Job drawing, mm, ordinate dimensions from the low corner. One solid piece. Give positions to 0.01 mm unless a question says otherwise; leave off trailing zeros. Write each loop counter-clockwise with the first axis right and the second up, starting at its lowest first coordinate (ties: lowest second). Pieces come first, ordered by that corner, then holes. Notation, with made-up numbers: M 79,52.5 L 108,52.5 A27 cw 108,88.5 Z; hole C 34,6 d7. An arc over 180 degrees is marked long. Use a Markdown table: item, result.
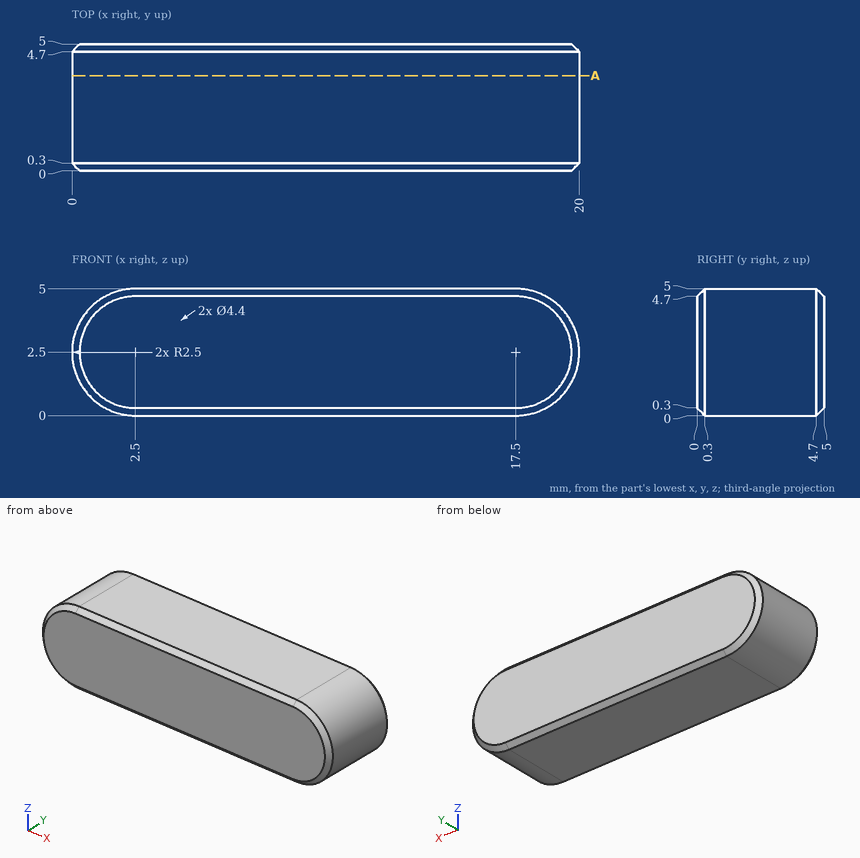
1. Drop flat-ended pins along their axis: P1, Ø3, axis at y = 1.5, z = 1, coming from the -X side; P2, Ø2, axis at y = 2.5, z = 4, coming from the -X side. Give the stop position or say it passes through.
Findings below:
| item | result |
|---|---|
| P1 | x = 0 |
| P2 | x = 0.05 |
2. Cut at A-A, the plane y = 3.75. Give the cut face in (x, z).
Findings below:
| item | result |
|---|---|
| outline | M 2.5,0 L 17.5,0 A2.5 ccw 17.5,5 L 2.5,5 A2.5 ccw Z |
3. Drill centre lines: L1, parallel to Z at x = 17.75, y = 0.7; L2, parallel to X at y = 3.15, z = 1.9; L3, parallel to X at y = 4.2, z = 2.05. Where is each one in solid material? Low to high.
Findings below:
| item | result |
|---|---|
| L1 | 0.01 to 4.99 |
| L2 | 0.07 to 19.93 |
| L3 | 0.04 to 19.96 |
